Here's how the part is built. I have some questions about the finished solid (model axes, mm). Round coordinates to 2 decimals unless told otherwise and drop trailing zeros. Write each loop counter-clockwise with the first axis right and the second up, starting at its lowest first coordinate (ties: lowest second). Pieces come first, ordered by that corner, then holes. Notation, with made-up numbers: (-13, 81) - (20, 81) arc R7 cw to (20, 88) - close; hole circle Ø2 at (-38.5, 54). An arc over 180 degrees is marked (long way). One line per question, with ' | ' between items. Start each with the question number.
(1) Imagine slicing it at B-B (x = 0). Write out the boundary of the cut face in (y, z).
(2) If I drill on L1, parallel to Y at x = -2.1, z = 0.1; L2, parallel to X at y = 154, z = 0.1; L3, parallel to X at y = 66.5, z = -0.65, over which ranges is the centre line in solid material (lowest first)?
(3) Imagine slicing it at C-C (y = 98). Write out the boundary of the cut face in (x, z).
(4) Will these pins go through, and if not, where does the flat tip stop? pin 1 (2 mm diameter, centred on x = 0, y = 53, fed in from +Z); pin 2 (1.5 mm diameter, centred on y = 124.5, z = 2, fed in from +X); pin 3 (1.5 mm diameter, centred on y = 113, z = -0.5, fed in from -X).
(5) Imagine slicing it at A-A (z = 0). Write out the boundary of the cut face in (x, y), plus the area to 3 significant figures.
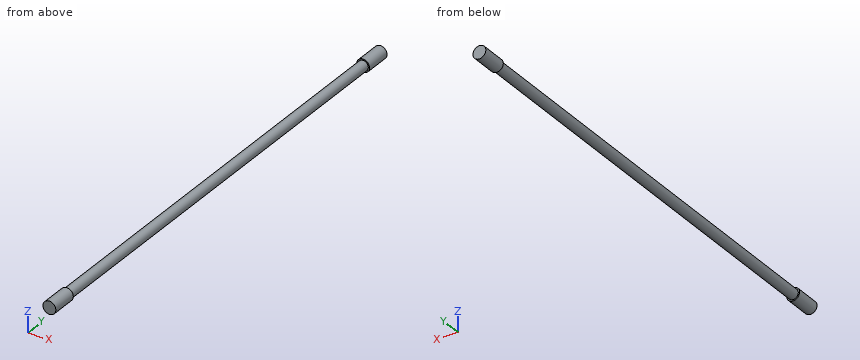
from build123d import *

# Parameters (mm, degrees)
F0_R     = 2.5
F1_DEPTH = 10
F2_R     = 2
F3_DEPTH = 170
F4_R     = 2.5
F4_R_2   = 2
F5_DEPTH = 10


with BuildPart() as f1:
    # F0 (on Front) → F1 (new body)
    with BuildSketch(Plane.XZ):
        Circle(F0_R)
    extrude(amount=-F1_DEPTH)

    # F2 (on face) → F3 (join)
    with BuildSketch(Plane(origin=(0, 10, 0), x_dir=(-1, 0, 0), z_dir=(0, 1, 0))):
        Circle(F2_R)
    extrude(amount=F3_DEPTH)

    # F4 (on face) → F5 (join)
    with BuildSketch(Plane(origin=(0, 180, 0), x_dir=(-1, 0, 0), z_dir=(0, 1, 0))):
        Circle(F4_R)
        Circle(F4_R_2, mode=Mode.SUBTRACT)
        Circle(F4_R_2)
    extrude(amount=F5_DEPTH)


solid = f1.part
Check sheet entries:
1) outline: (0, -2.5) - (10, -2.5) - (10, -2) - (180, -2) - (180, -2.5) - (190, -2.5) - (190, 2.5) - (180, 2.5) - (180, 2) - (10, 2) - (10, 2.5) - (0, 2.5) - close
2) L1: 0 to 10, 180 to 190 | L2: -2 to 2 | L3: -1.89 to 1.89
3) outline: circle Ø4 at (0, 0)
4) pin 1: z = 2 | pin 2: x = 1.56 | pin 3: x = -2
5) outline: (-2.5, 0) - (2.5, 0) - (2.5, 10) - (2, 10) - (2, 180) - (2.5, 180) - (2.5, 190) - (-2.5, 190) - (-2.5, 180) - (-2, 180) - (-2, 10) - (-2.5, 10) - close | area: 780 mm^2
